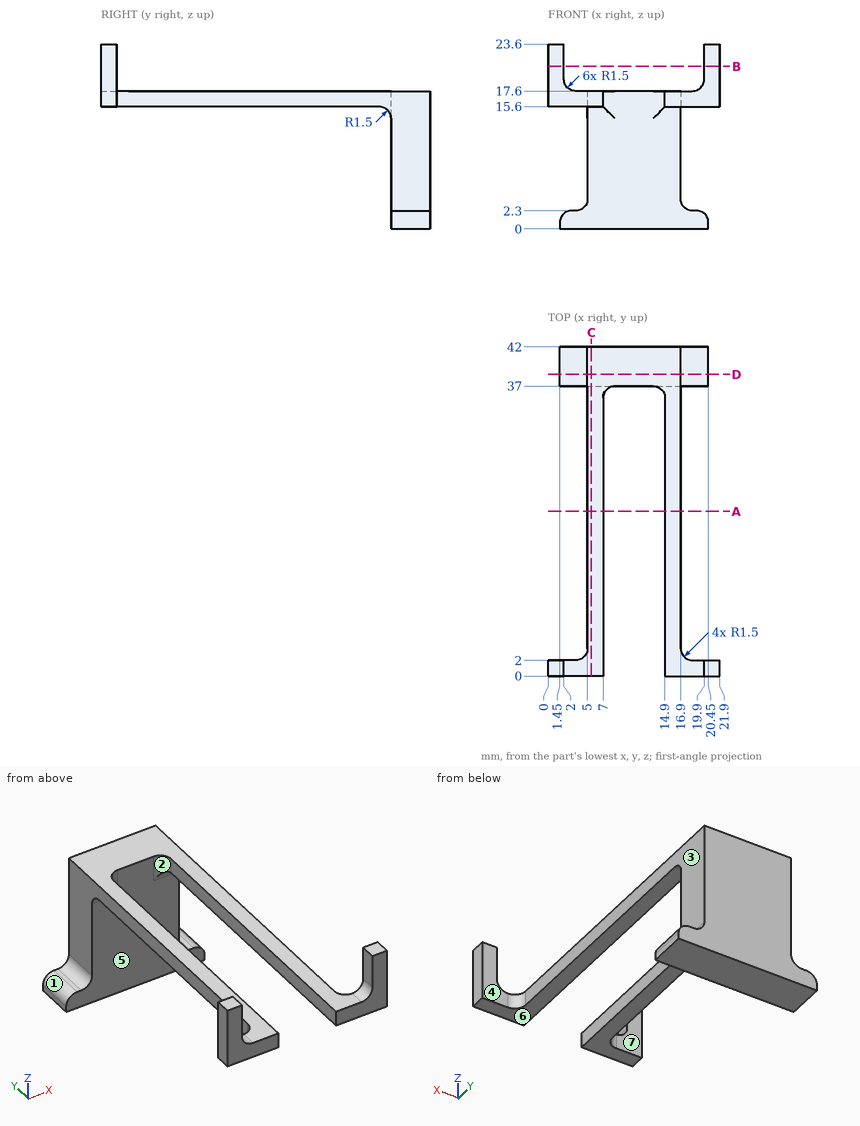
The drawing under review shows one solid part. Ordinate dimensions are in mm from its lowest x, y, z. A direction names the side the tool comes from. Round coordinates to 2 decimals unless told otherwise and drop trailing zeros. Loops run counter-clockwise (first coordinate to the right, second up) from the corner with the lowest first, then second, coordinate; pieces in that order, holes last. Notation, with made-up numbers: (53, 75) -> (65, 75) arc R21 ccw to (65, 85) -> close; hole circle Ø6 at (0, 67). An arc over 180 degrees is marked (long way). Answer in a Markdown table with one row per item.
1) For pin 1 Ø1.8 at (x, z) = (2, 20.5) entering from +Y; pin 2 Ø0.6 at (x, y) = (3, 40) entering from +Z; pin 3 Ø12 at (x, y) = (13, 16) entering from +Z, all flat-tipped, find the tip position at first contact; note any pin that passes through.
Taken from the geometry:
| item | result |
|---|---|
| pin 1 | stops at y = 2 |
| pin 2 | stops at z = 2.3 |
| pin 3 | stops at z = 17.6 |
2) Consider section A-A, the plane y = 21. Write out the cut boundary in (x, z), plus the area to 3 significant figures.
Taken from the geometry:
| item | result |
|---|---|
| outline | (5, 15.6) -> (7, 15.6) -> (7, 17.6) -> (5, 17.6) -> close; (14.9, 15.6) -> (16.9, 15.6) -> (16.9, 17.6) -> (14.9, 17.6) -> close |
| area | 8.00 mm² |
3) Consider section C-C, the plane x = 5.5. Write out the cut boundary in (y, z).
Taken from the geometry:
| item | result |
|---|---|
| outline | (0, 15.6) -> (35.5, 15.6) arc R1.5 cw to (37, 14.1) -> (37, 0) -> (42, 0) -> (42, 17.6) -> (0, 17.6) -> close |
4) Tool access review of the marked faces 4, 5, 6 and 7: name each direction out of +Z, -Z, +X, -X, +Y, -Y from which nothing blocks a thin tool from reaching the whole face with its end or side.
Taken from the geometry:
| item | result |
|---|---|
| face 4 | +Z, -Z, +X, +Y |
| face 5 | -Z, -Y |
| face 6 | -Z, +X, -X, -Y |
| face 7 | +Z, -Z, -X, +Y |
5) Consider section B-B, the plane z = 20.75. Write out the cut boundary in (x, y), plus the area to 3 significant figures.
Taken from the geometry:
| item | result |
|---|---|
| outline | (0, 0) -> (2, 0) -> (2, 2) -> (0, 2) -> close; (19.9, 0) -> (21.9, 0) -> (21.9, 2) -> (19.9, 2) -> close |
| area | 8.00 mm² |
6) Draft analysis for pull direction X (two halves, no side actions). For the marked faces 1, 2 and 3, state which applies: pulls with the +X half, pulls with the -X half, needs draft (parallel to the pull), parting line crosses it, or undercut.
Taken from the geometry:
| item | result |
|---|---|
| face 1 | pulls with the -X half |
| face 2 | undercut |
| face 3 | pulls with the +X half |
7) Consider section D-D, the plane y = 38.5. Write out the cut boundary in (x, z).
Taken from the geometry:
| item | result |
|---|---|
| outline | (1.45, 0) -> (20.45, 0) -> (20.45, 0.8) arc R1.5 ccw to (18.95, 2.3) -> (18.4, 2.3) arc R1.5 cw to (16.9, 3.8) -> (16.9, 17.6) -> (5, 17.6) -> (5, 3.8) arc R1.5 cw to (3.5, 2.3) -> (2.95, 2.3) arc R1.5 ccw to (1.45, 0.8) -> close |
8) Wall thickness on line 1 along Y through (x, z) = (13, 11.5); line 2 along X through (y, z) = (24.5, 17.25); line 3 along Z through (x, y) = (14.25, 39.5): over which ranges is each line inside the solid? List them lowest first.
Taken from the geometry:
| item | result |
|---|---|
| line 1 | y = 37 to 42 |
| line 2 | x = 5 to 7, 14.9 to 16.9 |
| line 3 | z = 0 to 17.6 |
